For this review, take the finished solid that the model builds, in its own axes (mm). Face numbers are marked on the shaded views. A direction names the side the tool comes from. Round coordinates to 2 decimals unless told otherwise and drop trailing zeros. Loops run counter-clockwise (first coordinate to the right, second up) from the corner with the lowest first, then second, coordinate; pieces in that order, holes last.
1. Consider section C-C on y = 49. State the section outline as (x, z) points.
2. Consider section D-D on x = -6. State how many separate pieces and enclosed holes the cut face has, then the cut area to 3 significant figures.
3. Clearance check with flat-ended pins moving along their axes: pin 1 Ø3 at (x, y) = (0, -23.75) entering from +Z; pin 2 Ø1.5 at (x, y) = (2.5, 67.5) entering from +Z; pin 3 Ø4 at (x, y) = (-19.5, 11) entering from -Z; pin 4 Ø3 at (x, y) = (11.5, 47) entering from +Z. State where each tip first meets the part, or that it passes through.
4. Consider section A-A on y = -23.75. State the section outline as (x, z) points.
5. To check wall thickness, follow line 1 along X through (y, z) = (27.9, -23.75); line 2 along Y through (x, z) = (0, -88.25); line 3 along Z through (x, y) = (-20, 67.05). State the ranges of each line that lie inside material, in increasing order.
6. Consider section B-B on y = 32. State the section outline as (x, z) points, then the cut area to 3 significant figures.
7. Tool access review of the marked faces 1, 2, 3, 4 and 5: name each direction out of +Z, -Z, +X, -X, +Y, -Y from which nothing blocks a thin tool from reaching the whole face with its end or side.
8. Draft analysis for pull direction Z (two halves, no side actions). For the marked faces 6, 7 and 8, state which applies: released by +Z, released by -Z, zero draft, split by the parting line, or undercut.
from build123d import *

# Parameters (mm, degrees)
SKETCH2_R                = 12.5
SKETCH2_R_2              = 10
BOSS_EXTRUDE1_START      = -5
SKETCH3_R                = 28.75
SKETCH3_R_2              = 10
BOSS_EXTRUDE1_DEPTH      = 5
HOLE1_D                  = 5
HOLE1_DEPTH              = 5
CIRPATTERN1_COUNT        = 4
SKETCH6_W                = 50
SKETCH6_H                = 50
SKETCH6_R                = 10
BOSS_EXTRUDE2_DEPTH      = 5
FILLET1_R                = 5
HOLE2_D                  = 5
BOSS_EXTRUDE3_REACH      = 120.882
BOSS_EXTRUDE3_END_RADIUS = 12.5
SKETCH9_R                = 10
HOLE3_REACH              = 120.882
HOLE3_BORE_R             = 7.5
SKETCH13_R               = 7.5
SKETCH13_R_2             = 2.5
BOSS_EXTRUDE4_DEPTH      = 3.75
BOSS_EXTRUDE5_REACH      = 135.902
BOSS_EXTRUDE5_END_RADIUS = 12.5
SKETCH14_R               = 10
HOLE4_REACH              = 135.902
HOLE4_BORE_R             = 7.5


with BuildPart() as part:
    # Sweep1: sweep along a path in Sketch1
    with BuildLine(Plane(origin=(0, 0, 0), x_dir=(0, 0, -1), z_dir=(1, 0, 0))) as sweep1_path:
        Line((0, 0), (56.25, 0))
        ThreePointArc((56.25, 0), (69.508252147, 5.491747853), (75, 18.75))
        Line((75, 18.75), (75, 68.75))
    # Sketch2 → Sweep1 (sweep)
    with BuildSketch(Plane.XY):
        Circle(SKETCH2_R)
        Circle(SKETCH2_R_2, mode=Mode.SUBTRACT)
    sweep(path=sweep1_path.line)

    # Sketch3 → Boss-Extrude1 (add)
    with BuildSketch(Plane.XY.offset(BOSS_EXTRUDE1_START)):
        Circle(SKETCH3_R)
        with Locations(Location((0, 0, 0), (0, 0, 270))):
            Circle(SKETCH3_R_2, mode=Mode.SUBTRACT)
    extrude(amount=BOSS_EXTRUDE1_DEPTH)

    # Hole1
    with Locations(Plane.XY):
        with Locations((23.75, 0)):
            hole1 = Hole(HOLE1_D / 2, depth=HOLE1_DEPTH)

    # CirPattern1: Hole1 ×4 about axis
    cirpattern1_axis = Axis((0, 0, 0), (0, 0, 1))
    for i in range(1, CIRPATTERN1_COUNT):
        add(hole1.rotate(cirpattern1_axis, i * 360 / CIRPATTERN1_COUNT), mode=Mode.SUBTRACT)

    # Sketch6 → Boss-Extrude2 (add)
    with BuildSketch(Plane(origin=(0, 68.75, 0), x_dir=(1, 0, 0), z_dir=(0, 1, 0))):
        with Locations((0, 75)):
            Rectangle(SKETCH6_W, SKETCH6_H)
        with Locations((0, 75)):
            Circle(SKETCH6_R, mode=Mode.SUBTRACT)
    extrude(amount=-BOSS_EXTRUDE2_DEPTH)

    # Fillet1
    fillet1_edges = [part.edges().sort_by_distance(p)[0] for p in [
        (25, 66.25, -100),
        (25, 66.25, -50),
        (-25, 66.25, -50),
        (-25, 66.25, -100),
    ]]
    fillet(fillet1_edges, radius=FILLET1_R)

    # Hole2 (through all)
    with Locations(Plane(origin=(0, 68.75, 0), x_dir=(1, 0, 0), z_dir=(0, 1, 0))):
        with Locations((-20, 55), (20, 55), (20, 95), (-20, 95)):
            Hole(HOLE2_D / 2)

    # Boss-Extrude3: up to this cylinder (the profile starts outside it)
    boss_extrude3_end = Plane(origin=(0, 0, -23.75), z_dir=(0, 0, -1)) * Cylinder(BOSS_EXTRUDE3_END_RADIUS, 267.764, mode=Mode.PRIVATE)
    # Sketch9 → Boss-Extrude3 (add, up to the surface)
    with BuildSketch(Plane(origin=(0, 28.75, 0), x_dir=(1, 0, 0), z_dir=(0, 1, 0)), mode=Mode.PRIVATE) as boss_extrude3_sk1:
        with Locations(Location((0, 23.75, 0), (0, 0, 270))):
            Circle(SKETCH9_R)
    boss_extrude3_tool1 = extrude(boss_extrude3_sk1.sketch, amount=-BOSS_EXTRUDE3_REACH, mode=Mode.PRIVATE) - boss_extrude3_end
    add(boss_extrude3_tool1.solids().sort_by_distance((0, 28.75, -23.75))[0])

    # Hole3 bore → Hole3 (cut, up to next)
    with BuildSketch(Plane(origin=(0, 28.75, 0), x_dir=(1, 0, 0), z_dir=(0, 1, 0)), mode=Mode.PRIVATE) as hole3_sk1:
        with Locations((0, 23.75)):
            Circle(HOLE3_BORE_R)
    hole3_tool1 = extrude(hole3_sk1.sketch, amount=-HOLE3_REACH, mode=Mode.PRIVATE) & part.part
    add(hole3_tool1.solids().sort_by_distance((0, 28.75, -23.75))[0], mode=Mode.SUBTRACT)

    # Sketch13 → Boss-Extrude4 (add)
    with BuildSketch(Plane(origin=(0, 28.75, 0), x_dir=(1, 0, 0), z_dir=(0, 1, 0))):
        with BuildLine():
            Line((-21.875, 28.385124054), (-4.6875, 35.337810136))
            ThreePointArc((-4.6875, 35.337810136), (0, 36.25), (4.6875, 35.337810136))
            Line((4.6875, 35.337810136), (21.875, 28.385124054))
            ThreePointArc((21.875, 28.385124054), (25, 23.75), (21.875, 19.114875946))
            Line((21.875, 19.114875946), (4.6875, 12.162189864))
            ThreePointArc((4.6875, 12.162189864), (0, 11.25), (-4.6875, 12.162189864))
            Line((-4.6875, 12.162189864), (-21.875, 19.114875946))
            ThreePointArc((-21.875, 19.114875946), (-25, 23.75), (-21.875, 28.385124054))
        make_face()
        with Locations(Location((0, 23.75, 0), (0, 0, 270))):
            Circle(SKETCH13_R, mode=Mode.SUBTRACT)
        with Locations(Location((-20, 23.75, 0), (0, 0, 270))):
            Circle(SKETCH13_R_2, mode=Mode.SUBTRACT)
        with Locations(Location((20, 23.75, 0), (0, 0, 270))):
            Circle(SKETCH13_R_2, mode=Mode.SUBTRACT)
    extrude(amount=-BOSS_EXTRUDE4_DEPTH)

    # Boss-Extrude5: up to this cylinder (the profile starts outside it)
    boss_extrude5_end = Plane(origin=(0, 51.25, -75), z_dir=(0, 1, 0)) * Cylinder(BOSS_EXTRUDE5_END_RADIUS, 297.804, mode=Mode.PRIVATE)
    # Sketch14 → Boss-Extrude5 (add, up to the surface)
    with BuildSketch(Plane.XY.offset(-111.25), mode=Mode.PRIVATE) as boss_extrude5_sk1:
        with Locations(Location((0, 51.25, 0), (0, 0, 180))):
            Circle(SKETCH14_R)
    boss_extrude5_tool1 = extrude(boss_extrude5_sk1.sketch, amount=BOSS_EXTRUDE5_REACH, mode=Mode.PRIVATE) - boss_extrude5_end
    add(boss_extrude5_tool1.solids().sort_by_distance((0, 51.25, -111.25))[0])

    # Hole4 bore → Hole4 (cut, up to next)
    with BuildSketch(Plane(origin=(0, 0, -111.25), x_dir=(-1, 0, 0), z_dir=(0, 0, -1)), mode=Mode.PRIVATE) as hole4_sk1:
        with Locations((0, 51.25)):
            Circle(HOLE4_BORE_R)
    hole4_tool1 = extrude(hole4_sk1.sketch, amount=-HOLE4_REACH, mode=Mode.PRIVATE) & part.part
    add(hole4_tool1.solids().sort_by_distance((0, 51.25, -111.25))[0], mode=Mode.SUBTRACT)


solid = part.part
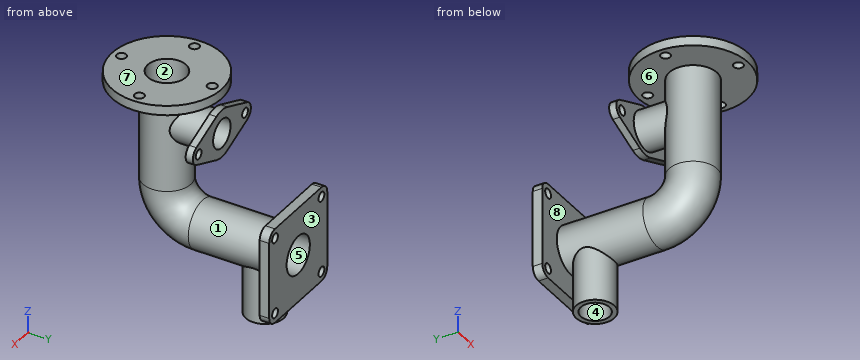
Resolved:
1. outline: (-9.74, -111.25) - (-7.15, -111.25) - (-7.15, -81.99) arc R10 cw (long way) to (7.15, -81.99) - (7.15, -111.25) - (9.74, -111.25) - (9.74, -82.83) arc R12.5 ccw (long way) to (-9.74, -82.83) - close
2. separate pieces: 4
2. enclosed holes: 0
2. area: 1,390 mm2
3. pin 1: passes through
3. pin 2: stops at z = -50
3. pin 3: stops at z = -5
3. pin 4: stops at z = -67.5
4. outline: (-16.2, -5) - (-2.5, -5) - (-2.5, 0) - (-16.2, 0) - close; (2.5, -5) - (16.2, -5) - (16.2, 0) - (2.5, 0) - close
5. line 1: x = -25 to -22.5, -17.5 to -7.5, 7.5 to 17.5, 22.5 to 25
5. line 2: y = 41.25 to 43.75, 58.75 to 61.25, 63.75 to 68.75
5. line 3: z = -100 to -97.5, -92.5 to -57.5, -52.5 to -50
6. outline: circle Ø25 at (0, -75); hole circle Ø20 at (0, -75)
6. area: 177 mm2
7. face 1: none
7. face 2: +Z
7. face 3: +Z, -Z, +X, -X, +Y
7. face 4: -Z
7. face 5: +Y
8. face 6: undercut
8. face 7: released by +Z
8. face 8: zero draft
